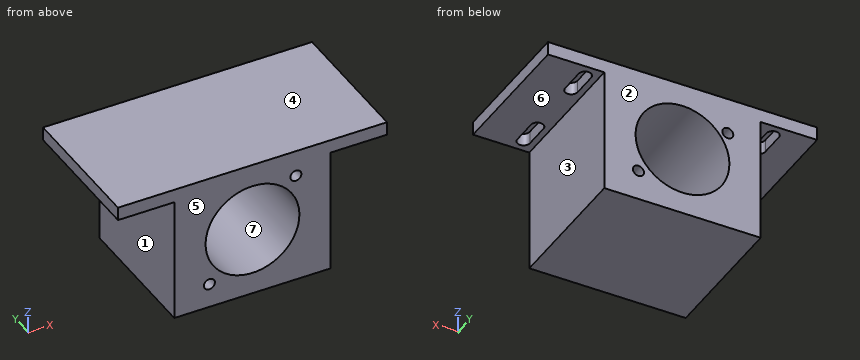
```python
from build123d import *

# Parameters (mm, degrees)
SKETCH_2_W             = 215
SKETCH_2_H             = 110
EXTRUDE_1_DEPTH        = 30
SKETCH_3_W             = 125
SKETCH_3_H             = 110
EXTRUDE_2_DEPTH        = 100
SKETCH_4_R             = 37.5
CUT_EXTRUDE_1_DEPTH    = 202.385823731
M10X1_25_2_AT_2_COUNT  = 2
M10X1_25_2_AT_2_PITCH  = 91.374081536
PATTERN_LINEAR_1_COUNT = 2
PATTERN_LINEAR_1_PITCH = 110
CUT_EXTRUDE_9_DEPTH    = 10
M10X1_25_4_D           = 8.8
M10X1_25_4_DEPTH       = 33.356213276
M10X1_25_4_TIP         = 2.643786724
SKETCH_28_W            = 215
SKETCH_28_H            = 19.25
CUT_EXTRUDE_11_DEPTH   = 110


with BuildPart() as part:
    # 草图2 → 凸台-拉伸1 (new body)
    with BuildSketch(Plane.XY):
        Rectangle(SKETCH_2_W, SKETCH_2_H)
    extrude(amount=-EXTRUDE_1_DEPTH)

    # 草图3 → 凸台-拉伸2 (add)
    with BuildSketch(Plane(origin=(0, 0, -30), x_dir=(-1, 0, 0), z_dir=(0, 0, -1))):
        Rectangle(SKETCH_3_W, SKETCH_3_H)
    extrude(amount=EXTRUDE_2_DEPTH)

    # 草图4 → 切除-拉伸1 (cut, through all)
    with BuildSketch(Plane(origin=(0, 55, 0), x_dir=(1, 0, 0), z_dir=(0, 1, 0))):
        with Locations(Location((0, 75, 0), (0, 0, 270))):
            Circle(SKETCH_4_R)
    extrude(amount=-CUT_EXTRUDE_1_DEPTH, mode=Mode.SUBTRACT)

    # 草图9 → M10x1.25 螺纹孔2 (revolve, cut)
    with BuildSketch(Plane(origin=(-36.193891144, 55, -48.668021168), x_dir=(0, 0, 1), z_dir=(1, 0, 0))):
        Polygon((0, 0), (0, 36), (4.4, 33.356213276), (4.4, 0), align=None)
    m10x1_25_2 = revolve(axis=Axis((-36.193891144, 61.35, -48.668021168), (0, -1, 0)), mode=Mode.SUBTRACT)

    # M10x1.25 螺纹孔2 at 2: M10x1.25 螺纹孔2 ×2
    with Locations(*[Vector(0.7813475015769275, 0, -0.624096211957334) * (i * M10X1_25_2_AT_2_PITCH) for i in range(1, M10X1_25_2_AT_2_COUNT)]):
        add(m10x1_25_2, mode=Mode.SUBTRACT)

    # 阵列(线性)1: M10x1.25 螺纹孔2 ×2
    with Locations(*[(0, i * PATTERN_LINEAR_1_PITCH, 0) for i in range(1, PATTERN_LINEAR_1_COUNT)]):
        add(m10x1_25_2, mode=Mode.SUBTRACT)

    # 阵列(线性)1 copy 1 sketch → 阵列(线性)1 copy 1 (revolve, cut)
    with BuildSketch(Plane(origin=(35.201019173, 165, -105.694239325), x_dir=(0, 0, 1), z_dir=(1, 0, 0))):
        Polygon((0, 0), (0, 36), (4.4, 33.356213276), (4.4, 0), align=None)
    revolve(axis=Axis((35.201019173, 171.35, -105.694239325), (0, -1, 0)), mode=Mode.SUBTRACT)

    # 草图14 → 切除-拉伸9 (cut)
    with BuildSketch(Plane(origin=(0, 0, -30), x_dir=(-1, 0, 0), z_dir=(0, 0, -1))):
        with BuildLine():
            Line((82.5, 45), (82.5, 25))
            ThreePointArc((82.5, 25), (77.5, 20), (72.5, 25))
            Line((72.5, 25), (72.5, 45))
            ThreePointArc((72.5, 45), (77.5, 50), (82.5, 45))
        make_face()
        with BuildLine():
            Line((-67.5, 45), (-67.5, 25))
            ThreePointArc((-67.5, 25), (-72.5, 20), (-77.5, 25))
            Line((-77.5, 25), (-77.5, 45))
            ThreePointArc((-77.5, 45), (-72.5, 50), (-67.5, 45))
        make_face()
        with BuildLine():
            Line((82.5, -25), (82.5, -45))
            ThreePointArc((82.5, -45), (77.5, -50), (72.5, -45))
            Line((72.5, -45), (72.5, -25))
            ThreePointArc((72.5, -25), (77.5, -20), (82.5, -25))
        make_face()
        with BuildLine():
            Line((-67.5, -25), (-67.5, -45))
            ThreePointArc((-67.5, -45), (-72.5, -50), (-77.5, -45))
            Line((-77.5, -45), (-77.5, -25))
            ThreePointArc((-77.5, -25), (-72.5, -20), (-67.5, -25))
        make_face()
    extrude(amount=-CUT_EXTRUDE_9_DEPTH, mode=Mode.SUBTRACT)

    # M10x1.25 螺纹孔4
    with Locations(Plane(origin=(0, -55, 0), x_dir=(-1, 0, 0), z_dir=(0, -1, 0))):
        with Locations((-34.688229548, 40.374629495), (34.423841578, 110.405583489)):
            Hole(M10X1_25_4_D / 2, depth=M10X1_25_4_DEPTH)
            with Locations((0, 0, -(M10X1_25_4_DEPTH + M10X1_25_4_TIP / 2))):  # 118° drill point
                Cone(0, M10X1_25_4_D / 2, M10X1_25_4_TIP, mode=Mode.SUBTRACT)

    # 草图28 → 切除-拉伸11 (cut)
    with BuildSketch(Plane.XZ.offset(55)):
        with Locations((0, -9.625)):
            Rectangle(SKETCH_28_W, SKETCH_28_H)
    extrude(amount=-CUT_EXTRUDE_11_DEPTH, mode=Mode.SUBTRACT)


solid = part.part
```
The model under review builds one solid part; all positions refer to its coordinate system, in mm. Face numbers are marked on the shaded views. A direction names the side the tool comes from. Give positions to 0.01 mm unless a question says otherwise; leave off trailing zeros. Order: outer loops, then holes, each group sorted by start corner. A loop starts at its lowest first (then second) coordinate and runs counter-clockwise, first axis right, second up. Notation, with made-up numbers: (-31, 72) - (22, 72) arc R19 cw to (22, 99) - close; hole circle Ø7 at (72.25, 73). An arc over 180 degrees is marked (long way). Use CSV: the item, a comma, the result in double quotes. Start each with the question number.
Q1. Clearance check with flat-ended pins moving along their axes: pin 1 Ø13.5 at (x, y) = (83, -8) entering from -Z; pin 2 Ø2 at (y, z) = (-33, -118) entering from +X; pin 3 Ø8 at (x, z) = (-34.42, -110.41) entering from -Y. State where each tip first meets the part, or that it passes through.
Q2. We need section D-D, the plane x = 72.5. Write out the cut boundary in (y, z).
Q3. Tool access review of the marked faces 1, 2 and 3: name each direction out of +Z, -Z, +X, -X, +Y, -Y from which nothing blocks a thin tool from reaching the whole face with its end or side.
Q4. We need section B-B, the plane y = 3.5. Write out the cut boundary in (x, z), and give its area (3 significant figures).
Q5. The part is to be moulded in two halves that separate along Z. For the marked faces 4, 5, 6 and 7, say which applies: +Z half, -Z half, draft (parallel to the pull), parting line (faces both ways), or undercut.
Q6. To check wall thickness, follow line 1 along X through (y, z) = (24, -50); line 2 along X through (y, z) = (35.5, -50.5); line 3 along Z through (x, y) = (33, -39.5). State the ranges of each line that lie inside material, in increasing order. Write a range as [from, to].
Q7. We need section A-A, the plane z = -75. Write out the cut boundary in (x, y), and give its area (3 significant figures).
Q8. We need section C-C, the plane x = 20. Write out the cut boundary in (y, z).
Outcome:
1,pin 1,"stops at z = -30"
1,pin 2,"stops at x = 62.5"
1,pin 3,"stops at y = -21.41"
2,outline,"(-55, -30) - (-50, -30) - (-50, -20) - (-20, -20) - (-20, -30) - (20, -30) - (20, -20) - (50, -20) - (50, -30) - (55, -30) - (55, -19.25) - (-55, -19.25) - close"
3,face 1,"-Z, -X, +Y, -Y"
3,face 2,"+Z, -Z, +X, -X, +Y"
3,face 3,"-Z, +X, +Y, -Y"
4,outline,"(-107.5, -30) - (-62.5, -30) - (-62.5, -130) - (62.5, -130) - (62.5, -30) - (107.5, -30) - (107.5, -19.25) - (-107.5, -19.25) - close; hole circle Ø75 at (0, -75)"
4,area,"10,400 mm^2"
5,face 4,"+Z half"
5,face 5,"draft"
5,face 6,"-Z half"
5,face 7,"undercut"
6,line 1,"x = [-62.5, -40.39], [-32, -27.95], [27.95, 62.5]"
6,line 2,"x = [-62.5, -40.19], [-32.19, -28.39], [28.39, 62.5]"
6,line 3,"z = [-130, -92.81], [-57.19, -44.44], [-36.31, -19.25]"
7,outline,"(-62.5, -55) - (-37.5, -55) - (-37.5, 55) - (-62.5, 55) - close; (37.5, -55) - (62.5, -55) - (62.5, 55) - (37.5, 55) - close"
7,area,"5,500 mm^2"
8,outline,"(-55, -130) - (55, -130) - (55, -106.72) - (-55, -106.72) - close; (-55, -43.28) - (55, -43.28) - (55, -19.25) - (-55, -19.25) - close"
